Input: part model. Units: mm. Frame: model coordinates. Coordinates: 2 decimals unless noted, no trailing zeros. Loops run counter-clockwise (first coordinate to the right, second up) from the corner with the lowest first, then second, coordinate; pieces in that order, holes last. Notation, with made-up numbers: (-28, -8) - (16, -8) arc R25 cw to (16, 29) - close; hole circle Ø3 at (13.25, 71.25). An arc over 180 degrees is marked (long way). Write item = value, one per line. Start each with the question number.
Autodesk Inventor part; units mm, degrees
ref_plane "YZ Plane" through (0, 0, 0) normal (1, 0, 0) x (0, 1, 0)
ref_plane "XZ Plane" through (0, 0, 0) normal (0, 1, 0) x (-1, 0, 0)
ref_plane "XY Plane" through (0, 0, 0) normal (0, 0, 1) x (1, 0, 0)
sketch "Sketch1" plane through (0, 0, 0) normal (0, 1, 0) x (-1, 0, 0)
  circle A0 centre (0, 0) radius 17.4625
  line L0 (0, 0) -> (17.4625, 0) construction
  dimension "d0" = 34.925
extrude "Extrusion1" add sketch "Sketch1" along normal blind 3.175
sketch "Sketch2" plane through (0, 3.175, 0) normal (0, 1, 0) x (1, 0, 0)
  circle A0 centre (0, 0) radius 2
  line L0 (0, 0) -> (-14.2875, 0) construction
  arc A1 (-12.8229, 3.4359) -> (-12.8229, -3.4359) centre (-9.525, 0) ccw
  circle A2 centre (0, 0) radius 7.5 construction
  circle A3 centre (-7.5, 0) radius 1.5
  circle A4 centre (3.75, -6.4952) radius 1.5
  circle A5 centre (3.75, 6.4952) radius 1.5
  dimension "d10" = 15
  dimension "d9" = 4
  dimension "d11" = 3
  dimension "d14" = 360
extrude "Extrusion2" cut sketch "Sketch2" against normal through all
chamfer "Chamfer1" distance 2 angle 45 3 edges at (-9, 3.175, 0) (2.25, 3.175, -6.4952) (2.25, 3.175, 6.4952)
chamfer "Chamfer2" distance 3.175 distance2 3.175 1 edges at (17.4625, 3.175, 0) measured on face at (10.0674, 3.175, 0)
properties part number "Hub Cap" material "Aluminum 6061"
Item 1: Cut plane B-B on y = 1.7. Return loops of the section in (x, z) (3 decimals), plus the area to 3 significant figures.
Item 2: Pin query (flat end, axial travel): pin 1 (4 mm diameter, centred on x = 3.75, z = -6.5, fed in from +Y); pin 2 (2.5 mm diameter, centred on x = -7.5, z = 0, fed in from -Y); pin 3 (1 mm diameter, centred on y = 0.5, z = -9.5, fed in from +X). Return the tip coordinate at first contact, or that it passes through.
Item 3: Pull-direction query (X, two-part tool) for faces 1 (the conical face through (3.14, 2.98, 14.14)), 2 (the flat face through (-4, 0, 0)), 3 (the conical face through (3.538, 1.3, 4.884)); classes: pulls with the +X half, pulls with the -X half, needs draft (parallel to the pull), parting line crosses it, or undercut.
Item 4: Ray query, line 1 (Z direction, x = 3.75, y = 0.3); line 2 (Z direction, x = 3.75, y = 0.85); line 3 (X direction, y = 1.75, z = -6). Return the intervals inside material, ascending.
Item 5: Cut plane A-A on z = 0. State how many separate pieces and enclosed holes the cut face has, plus the area to 3 significant figures.
Recorded:
q1.outline = circle Ø31.526 at (0, 0); hole circle Ø4.05 at (-7.5, 0); hole circle Ø4 at (0, 0); hole circle Ø4.05 at (3.75, -6.495); hole circle Ø4.05 at (3.75, 6.495)
q1.area = 729 mm²
q2.pin_1 = 1.68
q2.pin_2 = through
q2.pin_3 = 14.73
q3.face_1 = parting line crosses it
q3.face_2 = needs draft
q3.face_3 = undercut
q4.line_1 = -16.75 to -8, -5 to 5, 8 to 16.75
q4.line_2 = -16.18 to -8, -5 to 5, 8 to 16.18
q4.line_3 = -14.52 to 1.73, 5.77 to 14.52
q5.separate_pieces = 3
q5.enclosed_holes = 0
q5.area = 74.6 mm²
